The listing builds one solid part. Answer for the finished solid, in the listing's coordinates (mm). A direction names the side the tool comes from. Round coordinates to 2 decimals unless told otherwise and drop trailing zeros. Write each loop counter-clockwise with the first axis right and the second up, starting at its lowest first coordinate (ties: lowest second). Pieces come first, ordered by that corner, then holes.
(1) A cutting plane is placed at C-C, the plane x = -368. Give the vertices of the cut face in (y, z).
(2) The mould has two halves that part along Z. Classify faces 1 (the face through (89, 20, 133.35)), 2 (the face through (-151, 28, -158.75)), 3 (the face through (-169.514, 149.819, 155.853)): +Z half, -Z half, draft (parallel to the pull), parting line (faces both ways), or undercut.
(3) A cutting plane is placed at B-B, the plane y = 46.5. Give the vertices of the cut face in (x, z).
(4) For faces 4 (the face through (-309.94, 85.845, 155.853)), 5 (the face through (89, 20, -133.35)), 6 (the face through (73.145, 148.138, 155.853)), determine the directions among +Z, -Z, +X, -X, +Y, -Y from which every point of the face is accessible in a straight line to the end or side of a thin tool.
(5) A cutting plane is placed at A-A, the plane z = -21. Give the vertices of the cut face in (x, y), and give its area (3 significant figures).
(6) Each of these flat-tipped pins is pushed along its axis until it touches: pin 1 Ø10 at (y, z) = (-29, -81) entering from +X; pin 2 Ø12.5 at (x, z) = (95, -14) entering from +Y; pin 3 Ø12.5 at (x, z) = (75.5, -146.5) entering from +Y. Where does it stop, or does it pass through?
(7) Find the intervals of material crossed by probe 1 along X at (y, z) = (79, -22); probe 2 along Y at (x, z) = (-336.5, -42); probe 3 along Y at (x, z) = (-166, -97.5), in increasing order.
from build123d import *

# Parameters (mm, degrees)
BOSS_EXTRUDE1_DEPTH = 158.75
SKETCH2_W           = 25.4
SKETCH2_H           = 266.7
CUT_EXTRUDE1_DEPTH  = 139.7
FILLET1_R           = 10.16


with BuildPart() as part:
    # Sketch1 → Boss-Extrude1 (new, symmetric)
    with BuildSketch(Plane.XY):
        Polygon((-406.4, 88.9), (-406.4, -88.9), (101.6, -88.9), (101.6, 88.9), (76.2, 88.9), (76.2, 215.9), (-126.973642647, 215.9), (-215.9, 88.9), align=None)
    extrude(amount=BOSS_EXTRUDE1_DEPTH, both=True)

    # Sketch2 → Cut-Extrude1 (cut)
    with BuildSketch(Plane(origin=(0, 88.9, 0), x_dir=(1, 0, 0), z_dir=(0, 1, 0))):
        with Locations((88.9, 0)):
            Rectangle(SKETCH2_W, SKETCH2_H)
    extrude(amount=-CUT_EXTRUDE1_DEPTH, mode=Mode.SUBTRACT)

    # Fillet1
    fillet1_edges = [part.edges().sort_by_distance(p)[0] for p in [
        (-171.436821324, 152.4, 158.75),
        (-171.436821324, 152.4, -158.75),
        (-215.9, 88.9, 0),
        (-311.15, 88.9, 158.75),
        (-406.4, 88.9, 0),
        (-311.15, 88.9, -158.75),
        (76.2, 152.4, -158.75),
        (76.2, 152.4, 158.75),
        (-25.386821324, 215.9, -158.75),
        (-25.386821324, 215.9, 158.75),
        (76.2, 215.9, 0),
        (-126.973642647, 215.9, 0),
        (-406.4, 0, -158.75),
        (-406.4, 0, 158.75),
    ]]
    fillet(fillet1_edges, radius=FILLET1_R)


solid = part.part
Solutions:
1. outline: (-88.9, -158.75) - (78.74, -158.75) arc R10.16 ccw to (88.9, -148.59) - (88.9, 148.59) arc R10.16 ccw to (78.74, 158.75) - (-88.9, 158.75) - close
2. face 1: undercut
2. face 2: -Z half
2. face 3: +Z half
3. outline: (-406.4, -148.59) arc R10.16 ccw to (-396.24, -158.75) - (101.6, -158.75) - (101.6, -133.35) - (76.2, -133.35) - (76.2, 133.35) - (101.6, 133.35) - (101.6, 158.75) - (-396.24, 158.75) arc R10.16 ccw to (-406.4, 148.59) - close
4. face 4: +Z, -X, +Y
4. face 5: +X, +Y
4. face 6: +Z, +X, +Y
5. outline: (-406.4, -88.9) - (101.6, -88.9) - (101.6, -50.8) - (76.2, -50.8) - (76.2, 205.74) arc R10.16 ccw to (66.04, 215.9) - (-121.68, 215.9) arc R10.16 ccw to (-130.01, 211.57) - (-212.87, 93.23) arc R10.16 cw to (-221.19, 88.9) - (-396.24, 88.9) arc R10.16 ccw to (-406.4, 78.74) - close
5. area: 118,000 mm2
6. pin 1: stops at x = 76.2
6. pin 2: stops at y = -50.8
6. pin 3: stops at y = 215.38
7. probe 1: x = -406.4 to 76.2
7. probe 2: y = -88.9 to 88.9
7. probe 3: y = -88.9 to 160.16
